Design review of the part shown in the three views and the two pictorial views. Dimensions are in mm from the part's minimum x, y and z. A direction names the side the tool comes from. Coordinates: 2 decimals unless noted, no trailing zeros. Order: outer loops, then holes, each group sorted by start corner. A loop starts at its lowest first (then second) coordinate and runs counter-clockwise, first axis right, second up. Notation, with made-up numbers: (70, -4.5) - (100, -4.5) arc R17 cw to (100, 2.5) - close; hole circle Ø6 at (23, 75). An arc over 180 degrees is marked (long way). One line per item, written item: value. Start each with the question number.
(1) To check wall thickness, follow line 1 along Z through (x, y) = (23, 6.75); line 2 along X through (y, z) = (12.25, 9.5); line 3 along X through (y, z) = (10.75, 17). State the ranges of each line that lie inside material, in increasing order.
(2) Mouldability with a two-part tool opening along Z and no side actions: class the marked faces 4, 5 and 6 as released by +Z, released by -Z, zero draft, split by the parting line, or undercut.
(3) Consider section B-B on z = 10. Write out the cut boundary in (x, y).
(4) Consider section A-A on y = 2.75. Write out the cut boundary in (x, z).
(5) Consider section D-D on z = 6. Write out the cut boundary in (x, y), then the cut area to 3 significant figures.
(6) For the marked faces 1, 2 and 3, list the 3-axis set-ups (+Z, -Z, +X, -X, +Y, -Y) from which the entire face can be reached by the end or side of a thin tool; tool diameter is ignored.
(7) Clearance check with flat-ended pins moving along their axes: pin 1 (1.1 mm diameter, centred on y = 8.5, z = 10, fed in from +X); pin 2 (7 mm diameter, centred on x = 35.5, y = 2.5, fed in from +Z); pin 3 (0.6 mm diameter, centred on x = 49, y = 12, fed in from -Z). State where each tip first meets the part, or that it passes through.
(8) Consider section C-C on x = 9.5. Write out the cut boundary in (y, z).
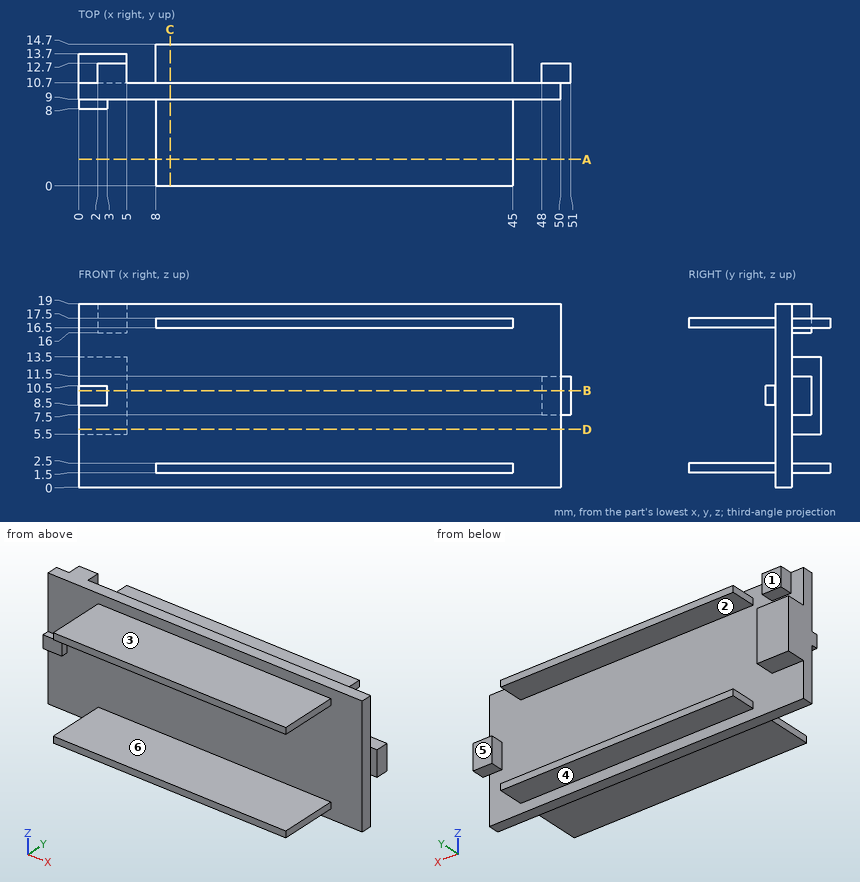
Geometry check:
1. line 1: z = 1.5 to 2.5, 16.5 to 17.5
1. line 2: x = 0 to 5, 48 to 51
1. line 3: x = 2 to 5, 8 to 45
2. face 4: released by -Z
2. face 5: zero draft
2. face 6: undercut
3. outline: (0, 8) - (3, 8) - (3, 9) - (50, 9) - (50, 10.7) - (51, 10.7) - (51, 12.7) - (48, 12.7) - (48, 10.7) - (5, 10.7) - (5, 13.7) - (0, 13.7) - close
4. outline: (8, 1.5) - (45, 1.5) - (45, 2.5) - (8, 2.5) - close; (8, 16.5) - (45, 16.5) - (45, 17.5) - (8, 17.5) - close
5. outline: (0, 9) - (50, 9) - (50, 10.7) - (5, 10.7) - (5, 13.7) - (0, 13.7) - close
5. area: 100 mm^2
6. face 1: +Z, -X, +Y
6. face 2: +X, +Y
6. face 3: +Z, +X, -X, -Y
7. pin 1: stops at x = 50
7. pin 2: stops at z = 17.5
7. pin 3: stops at z = 7.5
8. outline: (0, 1.5) - (9, 1.5) - (9, 0) - (10.7, 0) - (10.7, 1.5) - (14.7, 1.5) - (14.7, 2.5) - (10.7, 2.5) - (10.7, 16.5) - (14.7, 16.5) - (14.7, 17.5) - (10.7, 17.5) - (10.7, 19) - (9, 19) - (9, 17.5) - (0, 17.5) - (0, 16.5) - (9, 16.5) - (9, 2.5) - (0, 2.5) - close
